```python
from build123d import *

# Parameters (mm, degrees)
SKETCH4_W               = 1.524
SKETCH4_H               = 9.039794808
CUT_EXTRUDE2_DEPTH      = 1.016
SKETCH9_R               = 2.159
CUT_EXTRUDE3_DEPTH      = 4.9624
CUT_EXTRUDE3_DEPTH_BACK = 4.9624


with BuildPart() as part:
    # Sketch3 → Revolve1 (revolve)
    with BuildSketch(Plane.XY):
        Polygon((3.423584633, 13.716), (3.9624, 13.177184633), (3.9624, 0.538815367), (3.423584633, 0), (0, 0), (0, 13.716), align=None)
    revolve(axis=Axis((0, 0, 0), (0, 1, 0)))

    # Sketch4 → Cut-Extrude2 (cut)
    with BuildSketch(Plane(origin=(0, 13.716, 0), x_dir=(1, 0, 0), z_dir=(0, 1, 0))):
        with Locations((0, -0.098453211)):
            Rectangle(SKETCH4_W, SKETCH4_H)
    extrude(amount=-CUT_EXTRUDE2_DEPTH, mode=Mode.SUBTRACT)

    # Sketch9 → Cut-Extrude3 (cut, two sides)
    with BuildSketch(Plane.XY) as cut_extrude3_sk:
        with Locations((0, 6.858)):
            Circle(SKETCH9_R)
    extrude(amount=CUT_EXTRUDE3_DEPTH, mode=Mode.SUBTRACT)
    extrude(cut_extrude3_sk.sketch, amount=-CUT_EXTRUDE3_DEPTH_BACK, mode=Mode.SUBTRACT)


solid = part.part
```
Could you check a few things on this model? Use its own coordinates, in mm. A direction names the side the tool comes from. Coordinates: 2 decimals unless noted, no trailing zeros. Write each loop counter-clockwise with the first axis right and the second up, starting at its lowest first coordinate (ties: lowest second). Pieces come first, ordered by that corner, then holes. Notation, with made-up numbers: (-30.5, -30.75) -> (-16.5, -30.75) arc R36 ccw to (-16.5, 5.25) -> close; hole circle Ø5 at (-11, 26). An arc over 180 degrees is marked (long way). Return JSON: item names as keys, results as strings.
(1) Imagine slicing it at C-C, the plane y = 8.75. Please give me the cut outline in (x, z).
Numbers:
{"outline": "(-1.04, -3.82) -> (-1.04, 3.82) arc R3.96 ccw to start; (1.04, -3.82) arc R3.96 ccw to (1.04, 3.82) -> close"}
(2) Imagine slicing it at B-B, the plane y = 10.25. Please give me the cut outline in (x, z), then the cut area to 3 significant figures.
Numbers:
{"outline": "circle Ø7.92 at (0, 0)", "area": "49.3 mm2"}
(3) I'm going to push flat-ended pins straight in: pin 1 (1.2 mm diameter, centred on x = 0.5, z = -1.5, fed in from +Y); pin 2 (1 mm diameter, centred on y = 2.5, z = -1.5, fed in from -X); pin 3 (1.5 mm diameter, centred on x = 2, y = 7.5, fed in from -Z). Where does each tip first touch, or does it pass through?
Numbers:
{"pin 1": "stops at y = 13.72", "pin 2": "stops at x = -3.83", "pin 3": "stops at z = -3.58"}
(4) Imagine slicing it at A-A, the plane x = 0. Please give me the cut outline in (y, z).
Numbers:
{"outline": "(0, -3.42) -> (0.54, -3.96) -> (4.7, -3.96) -> (4.7, 3.96) -> (0.54, 3.96) -> (0, 3.42) -> close; (9.02, -3.96) -> (12.7, -3.96) -> (12.7, 3.96) -> (9.02, 3.96) -> close"}
(5) Which directions (+Z, -Z, +X, -X, +Y, -Y) give clear straight access to the entire face, cutting with the end or side of a thin tool? Please do faces 1 (the flat face through (0.762, 13, 0)), 2 (the flat face through (2, 13.716, 0)).
Numbers:
{"face 1": "+Z, -Z, +Y", "face 2": "+Z, -Z, +X, -X, +Y"}
(6) We'd pull the mould along X, two halves only. Please class faces 3 (the conical face through (3.58, 13.56, 0.07)), 4 (the cylindrical face through (3.78, 6.77, -1.19)), 5 (the flat face through (0, 12.7, 0)): +X half, -X half, draft (parallel to the pull), parting line (faces both ways), or undercut.
Numbers:
{"face 3": "+X half", "face 4": "parting line", "face 5": "undercut"}
(7) I need wall thicknesses on L1, parallel to Y at x = 0, z = -0.8; L2, parallel to Z at x = -2, y = 5.5; L3, parallel to X at y = 8.25, z = 3.25. Which ranges of each line are inside material? Lowest first, please.
Numbers:
{"L1": "y = 0 to 4.7, 9.02 to 12.7", "L2": "z = -3.42 to 3.42", "L3": "x = -2.27 to -1.65, 1.65 to 2.27"}
